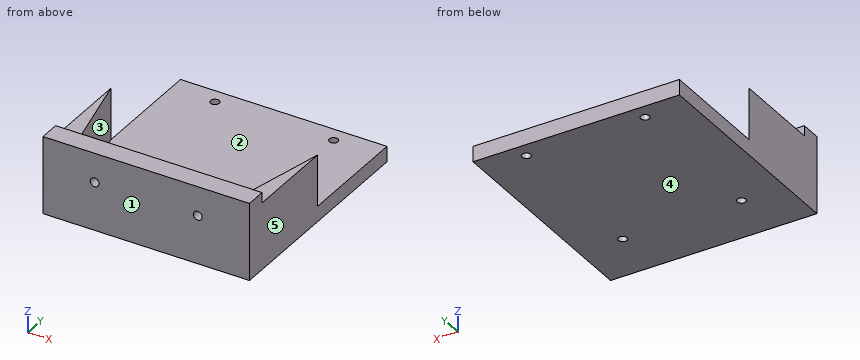
Solid Edge part; units mm, degrees
sketch "Sketch1" plane through (0, 0, 0) normal (0, 0, 1) x (1, 0, 0)
  line L0 (-40, -63) -> (40, -63)
  line L1 (40, -63) -> (40, 24)
  line L2 (40, 24) -> (-40, 24)
  line L3 (-40, 24) -> (-40, -63)
  circle A0 centre (-23, -43) radius 1.7
  circle A1 centre (23, -43) radius 1.7
  circle A2 centre (-23, 18) radius 1.7
  circle A3 centre (23, 18) radius 1.7
extrude "Protrusion1" add sketch "Sketch1" along normal blind 6
sketch "Sketch2" plane through (0, 0, 6) normal (0, 0, 1) x (1, 0, 0)
  line L0 (-40, -63) -> (40, -63)
  line L1 (40, -63) -> (40, -55)
  line L2 (40, -55) -> (-40, -55)
  line L3 (-40, -55) -> (-40, -63)
extrude "ExtrudedProtrusion_2" add sketch "Sketch2" along normal blind 24
sketch "Sketch3" plane through (0, 0, 6) normal (0, 0, 1) x (1, 0, 0)
  line L0 (-40, -55) -> (-32, -55)
  line L1 (-32, -55) -> (-40, -20)
  line L2 (-40, -20) -> (-40, -55)
extrude "ExtrudedProtrusion_3" add sketch "Sketch3" along normal blind 20
sketch "Sketch4" plane through (0, 0, 6) normal (0, 0, 1) x (1, 0, 0)
  line L0 (40, -55) -> (32, -55)
  line L1 (32, -55) -> (40, -20)
  line L2 (40, -20) -> (40, -55)
extrude "ExtrudedProtrusion_4" add sketch "Sketch4" along normal blind 20
sketch "Sketch5" plane through (0, -55, 0) normal (0, -1, 0) x (1, 0, 0)
  circle A0 centre (-20, 18.7) radius 1.7
  circle A1 centre (20, 18.7) radius 1.7
extrude "ExtrudedCutout_1" cut sketch "Sketch5" along normal blind 8
For this review, take the finished solid that the model builds, in its own axes (mm). Face numbers are marked on the shaded views. A direction names the side the tool comes from. Coordinates: 2 decimals unless noted, no trailing zeros. Loops run counter-clockwise (first coordinate to the right, second up) from the corner with the lowest first, then second, coordinate; pieces in that order, holes last. Notation, with made-up numbers: (84.5, 18.25) - (88.5, 18.25) arc R21 ccw to (88.5, 52.25) - close; hole circle Ø11 at (-5, -8.5). An arc over 180 degrees is marked (long way). Use a Markdown table: item, result. Add a question column.
Item 1: We need section D-D (y = 18). Give the boundary of the cut face in (x, z), and give its area (3 significant figures).
Item 2: For line 1 (Y direction, x = -23, z = 3.65); line 2 (Z direction, x = 20, y = -59.75); line 3 (Z direction, x = 1.5, y = -25), list the stretches that pass through material, from the lowest coordinate up.
Item 3: We need section A-A (x = 23). Give the boundary of the cut face in (y, z).
Item 4: Mouldability with a two-part tool opening along X and no side actions: class the marked faces 3, 4 and 5 as pulls with the +X half, pulls with the -X half, needs draft (parallel to the pull), parting line crosses it, or undercut.
Item 5: We need section C-C (x = -20). Give the boundary of the cut face in (y, z), and give its area (3 significant figures).
Item 6: Tool access review of the marked faces 1 and 2: name each direction out of +Z, -Z, +X, -X, +Y, -Y from which nothing blocks a thin tool from reaching the whole face with its end or side.
Item 7: We need section B-B (z = 18.7). Give the boundary of the cut face in (x, y).
Item 8: Insertion check: pin 1 Ø2 at (x, y) = (23, 18) entering from -Z; pin 2 Ø5.5 at (x, y) = (23, -43) entering from -Z; pin 3 Ø4 at (x, y) = (-36.5, -40) entering from +Z; pin 4 Ø6 at (x, z) = (-2, 17.5) entering from +Y. Each pin has a flat end and moves straight along its axis. Give the tip position at first contact, or say it passes through.
Results list:
| question | item | result |
|---|---|---|
| 1 | outline | (-40, 0) - (-24.7, 0) - (-24.7, 6) - (-40, 6) - close; (-21.3, 0) - (21.3, 0) - (21.3, 6) - (-21.3, 6) - close; (24.7, 0) - (40, 0) - (40, 6) - (24.7, 6) - close |
| 1 | area | 439 mm^2 |
| 2 | line 1 | y = -63 to -44.7, -41.3 to 16.3, 19.7 to 24 |
| 2 | line 2 | z = 0 to 17, 20.4 to 30 |
| 2 | line 3 | z = 0 to 6 |
| 3 | outline | (-63, 0) - (-44.7, 0) - (-44.7, 6) - (-55, 6) - (-55, 30) - (-63, 30) - close; (-41.3, 0) - (16.3, 0) - (16.3, 6) - (-41.3, 6) - close; (19.7, 0) - (24, 0) - (24, 6) - (19.7, 6) - close |
| 4 | face 3 | undercut |
| 4 | face 4 | needs draft |
| 4 | face 5 | pulls with the +X half |
| 5 | outline | (-63, 0) - (24, 0) - (24, 6) - (-55, 6) - (-55, 17) - (-63, 17) - close; (-63, 20.4) - (-55, 20.4) - (-55, 30) - (-63, 30) - close |
| 5 | area | 687 mm^2 |
| 6 | face 1 | +Z, -Z, +X, -X, -Y |
| 6 | face 2 | +Z, +Y |
| 7 | outline | (-40, -63) - (-21.7, -63) - (-21.7, -55) - (-32, -55) - (-40, -20) - close; (-18.3, -63) - (18.3, -63) - (18.3, -55) - (-18.3, -55) - close; (21.7, -63) - (40, -63) - (40, -20) - (32, -55) - (21.7, -55) - close |
| 8 | pin 1 | passes through |
| 8 | pin 2 | stops at z = 0 |
| 8 | pin 3 | stops at z = 26 |
| 8 | pin 4 | stops at y = -55 |
